Source: CAD feature listing. Evaluate the final solid. Frame: model axes, mm. Face numbers are marked on the shaded views. A direction names the side the tool comes from. Give positions to 0.01 mm unless a question says otherwise; leave off trailing zeros. Answer in a Markdown table with one row per item.
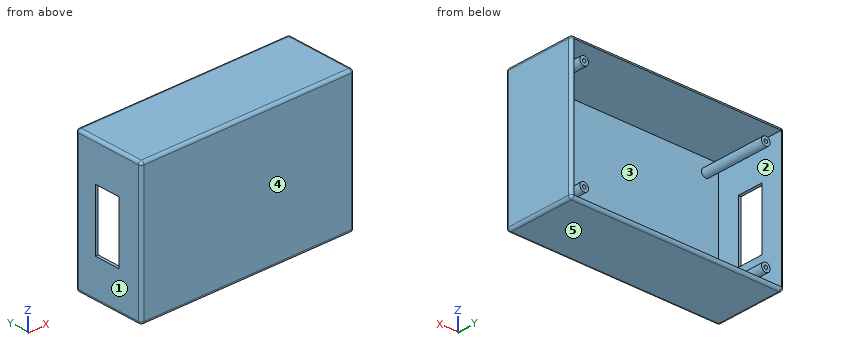
```python
from build123d import *

# Parameters (mm, degrees)
SKETCH1_W           = 149
SKETCH1_H           = 96.5
BOSS_EXTRUDE1_DEPTH = 50
SHELL2_T            = -2
SKETCH2_R           = 3
BOSS_EXTRUDE2_DEPTH = 46
SKETCH3_W           = 42.5
SKETCH3_H           = 18
CUT_EXTRUDE1_DEPTH  = 46
SKETCH4_R           = 1.25
CUT_EXTRUDE2_DEPTH  = 46
FILLET1_R           = 2


with BuildPart() as part:
    # Sketch1 → Boss-Extrude1 (new body)
    with BuildSketch(Plane(origin=(0, 0, 0), x_dir=(1, 0, 0), z_dir=(0, 1, 0))):
        Rectangle(SKETCH1_W, SKETCH1_H)
    extrude(amount=BOSS_EXTRUDE1_DEPTH)

    # Shell2
    shell2_openings = [part.faces().sort_by_distance(p)[0] for p in [
        (0, 50, 0),
    ]]
    offset(amount=SHELL2_T, openings=shell2_openings, kind=Kind.INTERSECTION)

    # Sketch2 → Boss-Extrude2 (add)
    with BuildSketch(Plane(origin=(0, 2, 0), x_dir=(1, 0, 0), z_dir=(0, 1, 0))):
        with Locations(Location((-63.5, 37.25, 0), (0, 0, 270))):
            Circle(SKETCH2_R)
        with Locations(Location((63.5, 37.25, 0), (0, 0, 270))):
            Circle(SKETCH2_R)
        with Locations(Location((63.5, -37.25, 0), (0, 0, 270))):
            Circle(SKETCH2_R)
        with Locations(Location((-63.5, -37.25, 0), (0, 0, 270))):
            Circle(SKETCH2_R)
    extrude(amount=BOSS_EXTRUDE2_DEPTH)

    # Sketch3 → Cut-Extrude1 (cut)
    with BuildSketch(Plane(origin=(-72.5, 0, 0), x_dir=(0, 0, -1), z_dir=(1, 0, 0))):
        with Locations((0, 26)):
            Rectangle(SKETCH3_W, SKETCH3_H)
    extrude(amount=-CUT_EXTRUDE1_DEPTH, mode=Mode.SUBTRACT)

    # Sketch4 → Cut-Extrude2 (cut)
    with BuildSketch(Plane(origin=(0, 48, 0), x_dir=(1, 0, 0), z_dir=(0, 1, 0))):
        with Locations(Location((63.5, -37.25, 0), (0, 0, 270))):
            Circle(SKETCH4_R)
        with Locations(Location((-63.5, 37.25, 0), (0, 0, 270))):
            Circle(SKETCH4_R)
        with Locations(Location((-63.5, -37.25, 0), (0, 0, 270))):
            Circle(SKETCH4_R)
        with Locations(Location((63.5, 37.25, 0), (0, 0, 270))):
            Circle(SKETCH4_R)
    extrude(amount=-CUT_EXTRUDE2_DEPTH, mode=Mode.SUBTRACT)

    # Fillet1
    fillet1_edges = [part.edges().sort_by_distance(p)[0] for p in [
        (-74.5, 50, 0),
        (0, 50, 48.25),
        (74.5, 50, 0),
        (0, 0, 48.25),
        (-74.5, 0, 0),
        (0, 0, -48.25),
        (74.5, 0, 0),
        (74.5, 25, 48.25),
        (-74.5, 25, 48.25),
        (-74.5, 25, -48.25),
        (74.5, 25, -48.25),
        (0, 50, -48.25),
    ]]
    fillet(fillet1_edges, radius=FILLET1_R - 0.0001)  # a hair under: the kernel refuses the full size


solid = part.part
```
(1) First-contact query: pin 1 Ø1 at (y, z) = (19.5, 20) entering from -X; pin 2 Ø6.5 at (x, z) = (63, -38) entering from +Y; pin 3 Ø0.6 at (x, z) = (-73.5, 7.5) entering from -Y. Flat tips, straight axial feed; report the tip coordinate or a pass-through.
A:
| item | result |
|---|---|
| pin 1 | stops at x = 72.5 |
| pin 2 | stops at y = 48 |
| pin 3 | stops at y = 0.13 |
(2) Section query A-A (y = 29.5). Give the number of separate pieces and of enclosed holes in the cut face, plus the area to 3 significant figures.
A:
| item | result |
|---|---|
| separate pieces | 5 |
| enclosed holes | 4 |
| area | 971 mm^2 |
(3) Pull-direction query (Z, two-part tool) for the marked faces 3, 4 and 5; classes: +Z half, -Z half, draft (parallel to the pull), parting line (faces both ways), or undercut.
A:
| item | result |
|---|---|
| face 3 | undercut |
| face 4 | draft |
| face 5 | -Z half |
(4) Ray query, probe 1 along X at (y, z) = (38, -37.25); probe 2 along Z at (x, y) = (-27, 42); probe 3 along Z at (x, y) = (63, 29). Return the intervals inside material, ascending.
A:
| item | result |
|---|---|
| probe 1 | x = -74.5 to -72.5, -66.5 to -64.75, -62.25 to -60.5, 60.5 to 62.25, 64.75 to 66.5, 72.5 to 74.5 |
| probe 2 | z = -48.25 to -46.25, 46.25 to 48.25 |
| probe 3 | z = -48.25 to -46.25, -40.21 to -38.4, -36.1 to -34.29, 34.29 to 36.1, 38.4 to 40.21, 46.25 to 48.25 |
(5) Access query for the marked faces 1 and 2. Directions: +Z, -Z, +X, -X, +Y, -Y. A direction counts if a zero-diameter tool reaches every point of the face in a straight line with its end or side. Return the directions, or none.
A:
| item | result |
|---|---|
| face 1 | +Z, -Z, -X, +Y, -Y |
| face 2 | +Y |
